The model under review builds one solid part; all positions refer to its coordinate system, in mm. Coordinates: 2 decimals unless noted, no trailing zeros. Write each loop counter-clockwise with the first axis right and the second up, starting at its lowest first coordinate (ties: lowest second). Pieces come first, ordered by that corner, then holes. Notation, with made-up numbers: (32, 64.25) -> (67, 64.25) arc R30 ccw to (67, 91.25) -> close; hole circle Ø10 at (1, -39). An arc over 180 degrees is marked (long way). Write each question's results on one line, items separated by ' | '.
```python
from build123d import *

# Parameters (mm, degrees)
SKIZZE1_W                       = 45
SKIZZE1_H                       = 45
SKIZZE1_R                       = 1.55
AUFSATZ_LINEAR_AUSTRAGEN1_DEPTH = 1.6
VERRUNDUNG1_R                   = 2


with BuildPart() as part:
    # Skizze1 → Aufsatz-Linear austragen1 (new body)
    with BuildSketch(Plane.XY):
        with Locations((22.5, 22.5)):
            Rectangle(SKIZZE1_W, SKIZZE1_H)
        with Locations((3, 42)):
            Circle(SKIZZE1_R, mode=Mode.SUBTRACT)
        with Locations((42, 42)):
            Circle(SKIZZE1_R, mode=Mode.SUBTRACT)
        with Locations((42, 3)):
            Circle(SKIZZE1_R, mode=Mode.SUBTRACT)
        with Locations((3, 3)):
            Circle(SKIZZE1_R, mode=Mode.SUBTRACT)
    extrude(amount=AUFSATZ_LINEAR_AUSTRAGEN1_DEPTH)

    # Verrundung1
    verrundung1_edges = [part.edges().sort_by_distance(p)[0] for p in [
        (0, 45, 0.8),
        (45, 45, 0.8),
        (45, 0, 0.8),
        (0, 0, 0.8),
    ]]
    fillet(verrundung1_edges, radius=VERRUNDUNG1_R)


solid = part.part
```
Q1. For line 1 (Y direction, x = 3, z = 0.6), list the stretches that pass through material, from the lowest coordinate up. Write a range as from..to.
Solution:
line 1: 0..1.45, 4.55..40.45, 43.55..45
Q2. Clearance check with a flat-ended pin moving along its axis: P1, Ø1.9, axis at x = 3, y = 42, coming from the +Z side. State where the tip first meets the part, or that it passes through.
Solution:
P1: through
Q3. Add section A-A (y = 3). Write out the cut boundary in (x, z).
Solution:
outline: (0, 0) -> (1.45, 0) -> (1.45, 1.6) -> (0, 1.6) -> close; (4.55, 0) -> (40.45, 0) -> (40.45, 1.6) -> (4.55, 1.6) -> close; (43.55, 0) -> (45, 0) -> (45, 1.6) -> (43.55, 1.6) -> close
Q4. Add section B-B (z = 0.3). Write out the cut boundary in (x, y).
Solution:
outline: (0, 2) arc R2 ccw to (2, 0) -> (43, 0) arc R2 ccw to (45, 2) -> (45, 43) arc R2 ccw to (43, 45) -> (2, 45) arc R2 ccw to (0, 43) -> close; hole circle Ø3.1 at (3, 3); hole circle Ø3.1 at (3, 42); hole circle Ø3.1 at (42, 3); hole circle Ø3.1 at (42, 42)
Q5. Draft analysis for pull direction X (two halves, no side actions). For faces 1 (the cylindrical face through (2.664, 40.487, 0.789)), 2 (the flat face through (45, 22, 1)), 3 (the flat face through (22, 45, 1)), state which applies: pulls with the +X half, pulls with the -X half, needs draft (parallel to the pull), parting line crosses it, or undercut.
Solution:
face 1: undercut | face 2: pulls with the +X half | face 3: needs draft
